```python
from build123d import *

# Parameters (mm, degrees)
SKETCH1_R           = 49.53
BOSS_EXTRUDE1_DEPTH = 3.175
SKETCH2_R           = 12.7
CUT_EXTRUDE1_DEPTH  = 3.175
SKETCH3_R           = 3.175
CUT_EXTRUDE2_DEPTH  = 3.175
SKETCH5_R           = 2.286
CUT_EXTRUDE3_DEPTH  = 3.175
CIRPATTERN1_COUNT   = 4
SKETCH6_R           = 2.286
CUT_EXTRUDE4_DEPTH  = 3.175
CIRPATTERN2_COUNT   = 4


with BuildPart() as part:
    # Sketch1 → Boss-Extrude1 (new body)
    with BuildSketch(Plane.XY):
        Circle(SKETCH1_R)
    extrude(amount=BOSS_EXTRUDE1_DEPTH)

    # Sketch2 → Cut-Extrude1 (cut)
    with BuildSketch(Plane.XY.offset(3.175)):
        with Locations((0, 27.432)):
            Circle(SKETCH2_R)
        with Locations((0, -27.432)):
            Circle(SKETCH2_R)
    extrude(amount=-CUT_EXTRUDE1_DEPTH, mode=Mode.SUBTRACT)

    # Sketch3 → Cut-Extrude2 (cut)
    with BuildSketch(Plane.XY.offset(3.175)):
        Circle(SKETCH3_R)
    extrude(amount=-CUT_EXTRUDE2_DEPTH, mode=Mode.SUBTRACT)

    # Sketch5 → Cut-Extrude3 (cut)
    with BuildSketch(Plane(origin=(0, 0, 0), x_dir=(-1, 0, 0), z_dir=(0, 0, -1))):
        with Locations((-12.886667534, -14.545332466)):
            Circle(SKETCH5_R)
    cut_extrude3 = extrude(amount=-CUT_EXTRUDE3_DEPTH, mode=Mode.SUBTRACT)

    # CirPattern1: Cut-Extrude3 ×4 about axis
    cirpattern1_axis = Axis((0, -27.432, 0), (0, 0, 1))
    for i in range(1, CIRPATTERN1_COUNT):
        add(cut_extrude3.rotate(cirpattern1_axis, i * 360 / CIRPATTERN1_COUNT), mode=Mode.SUBTRACT)

    # Sketch6 → Cut-Extrude4 (cut)
    with BuildSketch(Plane(origin=(0, 0, 0), x_dir=(-1, 0, 0), z_dir=(0, 0, -1))):
        with Locations((12.886667534, 14.545332466)):
            Circle(SKETCH6_R)
    cut_extrude4 = extrude(amount=-CUT_EXTRUDE4_DEPTH, mode=Mode.SUBTRACT)

    # CirPattern2: Cut-Extrude4 ×4 about axis
    cirpattern2_axis = Axis((0, 27.432, 0), (0, 0, 1))
    for i in range(1, CIRPATTERN2_COUNT):
        add(cut_extrude4.rotate(cirpattern2_axis, i * 360 / CIRPATTERN2_COUNT), mode=Mode.SUBTRACT)


solid = part.part
```
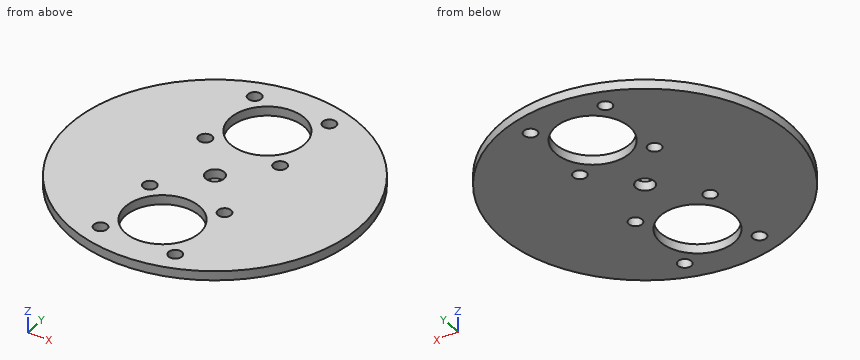
The model under review builds one solid part; all positions refer to its coordinate system, in mm. Coordinates: 2 decimals unless noted, no trailing zeros. Write each loop counter-clockwise with the first axis right and the second up, starting at its lowest first coordinate (ties: lowest second). Pieces come first, ordered by that corner, then holes.
1) Clearance check with flat-ended pins moving along their axes: pin 1 Ø2.5 at (x, y) = (12.89, -14.55) entering from -Z; pin 2 Ø1 at (x, z) = (-19.5, 2.5) entering from +Y; pin 3 Ø1.5 at (y, z) = (6, 0.5) entering from +X; pin 4 Ø1.5 at (x, z) = (-11.5, 2) entering from +Y. State where each tip first meets the part, or that it passes through.
2) We need section A-A on y = 0. State the section outline as (x, z) points (3 decimals), then the cut area to 3 significant figures.
3) We need section D-D on y = 35. State the section outline as (x, z) points (3 decimals).
4) To check wall thickness, follow probe 1 along Y at (x, z) = (0, 1.6) (3 decimals); probe 2 along Y at (x, z) = (9, 1.8); probe 3 along X at (y, z) = (-38.5, 2.65). State the ranges of each line that lie inside material, in increasing order.
5) We need section B-B on x = 0. State the section outline as (y, z) points (3 decimals), then the cut area to 3 significant figures.
6) We need section C-C on z = 1.55. Count the separate pieces of the cut face and the enclosed holes in it, then the cut area to 3 significant figures.
Answer list:
1. pin 1: passes through
1. pin 2: stops at y = 45.74
1. pin 3: stops at x = 49.25
1. pin 4: stops at y = 48.35
2. outline: (-49.53, 0) - (-3.175, 0) - (-3.175, 3.175) - (-49.53, 3.175) - close; (3.175, 0) - (49.53, 0) - (49.53, 3.175) - (3.175, 3.175) - close
2. area: 294 mm2
3. outline: (-35.046, 0) - (-10.199, 0) - (-10.199, 3.175) - (-35.046, 3.175) - close; (10.199, 0) - (35.046, 0) - (35.046, 3.175) - (10.199, 3.175) - close
4. probe 1: y = -49.53 to -40.132, -14.732 to -3.175, 3.175 to 14.732, 40.132 to 49.53
4. probe 2: y = -48.71 to -36.39, -18.47 to 18.47, 36.39 to 48.71
4. probe 3: x = -31.16 to -14.27, -11.5 to -6.23, 6.23 to 11.5, 14.27 to 31.16
5. outline: (-49.53, 0) - (-40.132, 0) - (-40.132, 3.175) - (-49.53, 3.175) - close; (-14.732, 0) - (-3.175, 0) - (-3.175, 3.175) - (-14.732, 3.175) - close; (3.175, 0) - (14.732, 0) - (14.732, 3.175) - (3.175, 3.175) - close; (40.132, 0) - (49.53, 0) - (49.53, 3.175) - (40.132, 3.175) - close
5. area: 133 mm2
6. separate pieces: 1
6. enclosed holes: 11
6. area: 6,530 mm2
